Verification items for the finished model (mm, model axes). Coordinates: 2 decimals unless noted, no trailing zeros. Loops run counter-clockwise (first coordinate to the right, second up) from the corner with the lowest first, then second, coordinate; pieces in that order, holes last. Notation, with made-up numbers: (55, 79) - (111, 79) arc R20 cw to (111, 118) - close; hole circle Ø6 at (55, 54.5). An arc over 180 degrees is marked (long way). One line per item, written item: value. Start each with the question number.
(1) Section check B-B (x = -117). Record the boundary of the cut face in (y, z), plus the area to 3 significant figures.
(2) Section check A-A (y = 0). Record the boundary of the cut face in (x, z).
(3) Section check C-C (z = 20). Record the boundary of the cut face in (x, y) (1 decimal).
(4) Thickness scan on probe 1 along Y at (x, z) = (-53, 13); probe 2 along X at (y, z) = (-2.25, 14); probe 3 along X at (y, z) = (3, 27.5). Record the ranges inside material, lowest first. Write a range as [from, to].
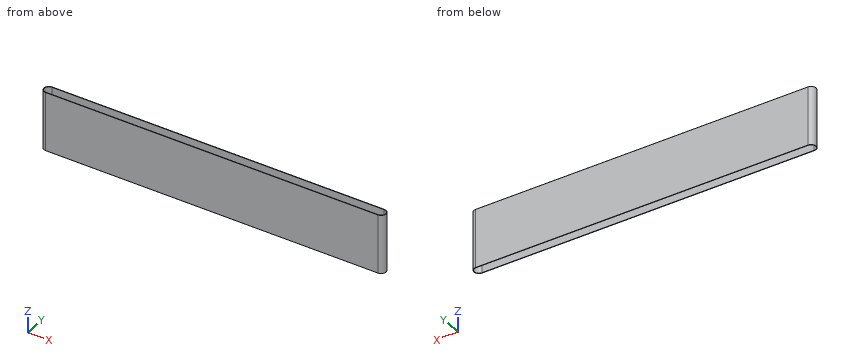
```python
from build123d import *

# Parameters (mm, degrees)
BOSS_EXTRUDE1_DEPTH = 50.673
FILLET1_R           = 0.127


with BuildPart() as part:
    # Sketch2 → Boss-Extrude1 (new body)
    with BuildSketch(Plane.XY):
        with BuildLine():
            Line((-142.875, 4.2545), (142.875, 4.2545))
            ThreePointArc((142.875, 4.2545), (147.1295, 0), (142.875, -4.2545))
            Line((142.875, -4.2545), (-142.875, -4.2545))
            ThreePointArc((-142.875, -4.2545), (-147.1295, 0), (-142.875, 4.2545))
        make_face()
        with BuildLine():
            ThreePointArc((142.875, -3.8735), (146.7485, 0), (142.875, 3.8735))
            Line((142.875, 3.8735), (-142.875, 3.8735))
            ThreePointArc((-142.875, 3.8735), (-146.7485, 0), (-142.875, -3.8735))
            Line((-142.875, -3.8735), (142.875, -3.8735))
        make_face(mode=Mode.SUBTRACT)
    extrude(amount=BOSS_EXTRUDE1_DEPTH)

    # Fillet1
    fillet1_edges = [part.edges().sort_by_distance(p)[0] for p in [
        (147.1295, 0, 0),
        (0, -4.2545, 0),
        (-147.1295, 0, 0),
        (0, 4.2545, 0),
        (0, -3.8735, 50.673),
        (0, 3.8735, 0),
        (-146.7485, 0, 0),
        (0, -3.8735, 0),
        (146.7485, 0, 0),
        (-146.7485, 0, 50.673),
        (0, 3.8735, 50.673),
        (0, 4.2545, 50.673),
        (-147.1295, 0, 50.673),
        (0, -4.2545, 50.673),
        (147.1295, 0, 50.673),
        (146.7485, 0, 50.673),
    ]]
    fillet(fillet1_edges, radius=FILLET1_R)


solid = part.part
```
Responses:
1. outline: (-4.25, 0.13) arc R0.13 ccw to (-4.13, 0) - (-4, 0) arc R0.13 ccw to (-3.87, 0.13) - (-3.87, 50.55) arc R0.13 ccw to (-4, 50.67) - (-4.13, 50.67) arc R0.13 ccw to (-4.25, 50.55) - close; (3.87, 0.13) arc R0.13 ccw to (4, 0) - (4.13, 0) arc R0.13 ccw to (4.25, 0.13) - (4.25, 50.55) arc R0.13 ccw to (4.13, 50.67) - (4, 50.67) arc R0.13 ccw to (3.87, 50.55) - close
1. area: 38.6 mm²
2. outline: (-147.13, 0.13) arc R0.13 ccw to (-147, 0) - (-146.88, 0) arc R0.13 ccw to (-146.75, 0.13) - (-146.75, 50.55) arc R0.13 ccw to (-146.88, 50.67) - (-147, 50.67) arc R0.13 ccw to (-147.13, 50.55) - close; (146.75, 0.13) arc R0.13 ccw to (146.88, 0) - (147, 0) arc R0.13 ccw to (147.13, 0.13) - (147.13, 50.55) arc R0.13 ccw to (147, 50.67) - (146.88, 50.67) arc R0.13 ccw to (146.75, 50.55) - close
3. outline: (-142.9, -4.3) - (142.9, -4.3) arc R4.3 ccw to (142.9, 4.3) - (-142.9, 4.3) arc R4.3 ccw to start; hole (-142.9, -3.9) - (142.9, -3.9) arc R3.9 ccw to (142.9, 3.9) - (-142.9, 3.9) arc R3.9 ccw to start
4. probe 1: y = [-4.25, -3.87], [3.87, 4.25]
4. probe 2: x = [-146.49, -146.03], [146.03, 146.49]
4. probe 3: x = [-145.89, -145.33], [145.33, 145.89]
